Design review of the part built by this model. Coordinates are the model's own, in mm. A direction names the side the tool comes from. Give positions to 0.01 mm unless a question says otherwise; leave off trailing zeros. Order: outer loops, then holes, each group sorted by start corner. A loop starts at its lowest first (then second) coordinate and runs counter-clockwise, first axis right, second up. Notation, with made-up numbers: (16.5, 66) - (29.5, 66) arc R24 cw to (29.5, 104) - close; hole circle Ø11 at (-17.75, 22). An arc over 180 degrees is marked (long way). Write each question's results on one line, items separated by ' | '. Start each with the question number.
```python
from build123d import *

# Parameters (mm, degrees)
SKETCH_1_W          = 45
SKETCH_1_H          = 45
EXTRUDE_1_DEPTH     = 20
SKETCH_2_W          = 41
SKETCH_2_H          = 41
CUT_EXTRUDE_1_DEPTH = 17
CUT_EXTRUDE_1_DRAFT = -2


with BuildPart() as part:
    # Эскиз1 → Бобышка-Вытянуть1 (new body)
    with BuildSketch(Plane.XY):
        Rectangle(SKETCH_1_W, SKETCH_1_H)
    extrude(amount=EXTRUDE_1_DEPTH)


with BuildPart() as cut_extrude_1_tool:
    # Эскиз2 → Вырез-Вытянуть1 (with draft: the straight prism first)
    with BuildSketch(Plane.XY.offset(20)):
        Rectangle(SKETCH_2_W, SKETCH_2_H)
    extrude(amount=-CUT_EXTRUDE_1_DEPTH)
    # Вырез-Вытянуть1: the draft: its side faces are tilted about the plane it starts from
    cut_extrude_1_sides = [cut_extrude_1_tool.faces().sort_by_distance(p)[0] for p in [
        (-20.5, 0, 11.5),
        (0, -20.5, 11.5),
        (20.5, 0, 11.5),
        (0, 20.5, 11.5),
    ]]
    draft(cut_extrude_1_sides, Plane.XY.offset(20), CUT_EXTRUDE_1_DRAFT)


with BuildPart() as part_1:
    add(part.part)

    # Вырез-Вытянуть1: cut by cut_extrude_1_tool
    add(cut_extrude_1_tool.part, mode=Mode.SUBTRACT)


solid = part_1.part
```
Q1. Insertion check: pin 1 Ø3 at (x, y) = (3.5, 2) entering from +Z; pin 2 Ø4 at (x, y) = (16, -4) entering from -Z. Each pin has a flat end and moves straight along its axis. Give the tip position at first contact, or say it passes through.
Q2. For line 1 (Y direction, x = -5, z = 13.25); line 2 (Z direction, x = -3, y = -9); line 3 (Y direction, x = -2, z = 4.5), list the stretches that pass through material, from the lowest coordinate up. Write a range as [from, to].
Q3. Add section A-A (z = 6). Give the boundary of the cut face in (x, y).
Q4. Add section B-B (x = -6). Give the boundary of the cut face in (y, z).
Q5. Machinability: for faces 1 (the flat face through (-22.5, 0, 10)), 2 (the flat face through (0, 0, 3)), which of the approach directions +Z, -Z, +X, -X, +Y, -Y give a long, thin tool a straight path to every point of the face, cutting with its end or side? Answer none if there is none.
Q6. Add section D-D (z = 10). Give the boundary of the cut face in (x, y), plus the area to 3 significant figures.
Verdict:
1) pin 1: stops at z = 3 | pin 2: stops at z = 0
2) line 1: y = [-22.5, -20.26], [20.26, 22.5] | line 2: z = [0, 3] | line 3: y = [-22.5, -19.96], [19.96, 22.5]
3) outline: (-22.5, -22.5) - (22.5, -22.5) - (22.5, 22.5) - (-22.5, 22.5) - close; hole (-20.01, -20.01) - (20.01, -20.01) - (20.01, 20.01) - (-20.01, 20.01) - close
4) outline: (-22.5, 0) - (22.5, 0) - (22.5, 20) - (20.5, 20) - (19.91, 3) - (-19.91, 3) - (-20.5, 20) - (-22.5, 20) - close
5) face 1: +Z, -Z, -X, +Y, -Y | face 2: +Z
6) outline: (-22.5, -22.5) - (22.5, -22.5) - (22.5, 22.5) - (-22.5, 22.5) - close; hole (-20.15, -20.15) - (20.15, -20.15) - (20.15, 20.15) - (-20.15, 20.15) - close | area: 401 mm2
